Verification items for the finished model (mm, model axes). Face numbers are marked on the shaded views. A direction names the side the tool comes from. Coordinates: 2 decimals unless noted, no trailing zeros. Order: outer loops, then holes, each group sorted by start corner. A loop starts at its lowest first (then second) coordinate and runs counter-clockwise, first axis right, second up. Notation, with made-up numbers: (62.5, 56) -> (94.5, 56) arc R17 ccw to (94.5, 81) -> close; hole circle Ø10 at (-22, -14.5). An arc over 180 degrees is marked (long way). Answer as CSV lines item,"result".
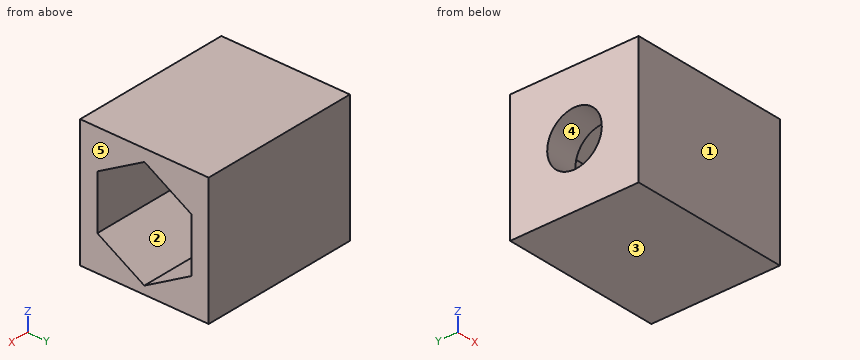
```python
from build123d import *

# Parameters (mm, degrees)
CYLINDER031_R              = 1.7
CYLINDER031_DEPTH          = 20
EXTRUDE004_DEPTH           = 9
EXTRUDE004_PLACEMENT_ANGLE = 90
BOX042_W                   = 10
BOX042_H                   = 8
BOX042_DEPTH               = 8


with BuildPart() as cylinder031:
    # Cylinder031 → Cylinder031 (new body)
    with BuildSketch(Plane(origin=(140, 9.74, 51.5), x_dir=(0, 0, -1), z_dir=(1, 0, 0))):
        Circle(CYLINDER031_R)
    extrude(amount=CYLINDER031_DEPTH)


with BuildPart() as extrude004:
    # Sketch004 → Extrude004 (new body)
    with BuildSketch(Plane.XY.offset(75)):
        Polygon((-29.694611, 6.813304), (-28.00073, 9.738351), (-29.686954, 12.667818), (-33.06706, 12.672239), (-34.760941, 9.747192), (-33.074716, 6.817725), align=None)
    extrude(amount=EXTRUDE004_DEPTH)


with BuildPart() as extrude004_1:
    # Extrude004 placement: moved
    add(extrude004.part.moved(Location((71, 0, 0))).rotate(Axis((71, 0, 0), (0, 1, 0)), EXTRUDE004_PLACEMENT_ANGLE))


with BuildPart() as cut050:
    # Box042 → Box042 (new body)
    with BuildSketch(Plane(origin=(144, 5.745, 27.5), x_dir=(1, 0, 0), z_dir=(0, 0, 1))):
        with Locations((5, 4)):
            Rectangle(BOX042_W, BOX042_H)
    extrude(amount=BOX042_DEPTH)

    # Cut049: cut Extrude004
    add(extrude004_1.part, mode=Mode.SUBTRACT)


with BuildPart() as cut050_1:
    # Cut049 placement: moved
    add(cut050.part.moved(Location((0, 0, 20))))

    # Cut050: cut Cylinder031
    add(cylinder031.part, mode=Mode.SUBTRACT)


solid = cut050_1.part
```
Item 1: Tool access check on the marked faces 1 and 2. Record the directions out of +Z, -Z, +X, -X, +Y, -Y that give a thin tool (end or side, any length) a straight path to the whole face; none if there is none.
Answer list:
face 1,"+Z, -Z, +X, -X, -Y"
face 2,"+X"
Item 2: Release check for a two-part mould opening along Z. For the marked faces 3, 4 and 5 record: +Z half, -Z half, draft (parallel to the pull), parting line (faces both ways), or undercut.
Answer list:
face 3,"-Z half"
face 4,"undercut"
face 5,"draft"
Item 3: Section check D-D, the plane z = 54. Record the boundary of the cut face in (x, y) (3 decimals), plus the area to 3 significant figures.
Answer list:
outline,"(144, 5.745) -> (154, 5.745) -> (154, 8.425) -> (146, 8.425) -> (146, 11.061) -> (154, 11.061) -> (154, 13.745) -> (144, 13.745) -> close"
area,"58.9 mm2"
Item 4: Section check B-B, the plane x = 145. Record the boundary of the cut face in (y, z) (3 decimals), plus the area to 3 significant figures.
Answer list:
outline,"(5.745, 47.5) -> (13.745, 47.5) -> (13.745, 55.5) -> (5.745, 55.5) -> close; hole circle Ø3.4 at (9.74, 51.5)"
area,"54.9 mm2"
Item 5: Section check C-C, the plane y = 10.5. Record the boundary of the cut face in (x, z) (3 decimals), plus the area to 3 significant figures.
Answer list:
outline,"(144, 47.5) -> (154, 47.5) -> (154, 48.439) -> (146, 48.439) -> (146, 49.979) -> (144, 49.979) -> close; (144, 53.021) -> (146, 53.021) -> (146, 54.325) -> (154, 54.325) -> (154, 55.5) -> (144, 55.5) -> close"
area,"26.8 mm2"
Item 6: Depth check by flat-ended pin: pin 1 Ø1.5 at (y, z) = (11.5, 50) entering from +X. Enter the tip coordinate at first touch or a pass-through.
Answer list:
pin 1,"x = 146"
Item 7: Section check A-A, the plane z = 52.5. Record the boundary of the cut face in (x, y) (1 decimal).
Answer list:
outline,"(144, 5.7) -> (154, 5.7) -> (154, 6.8) -> (146, 6.8) -> (146, 8.4) -> (144, 8.4) -> close; (144, 11.1) -> (146, 11.1) -> (146, 12.7) -> (154, 12.7) -> (154, 13.7) -> (144, 13.7) -> close"
Item 8: Thickness scan on line 1 (Y direction, x = 145.3, z = 51.5) (3 decimals); line 2 (Y direction, x = 146.75, z = 52.75) (3 decimals); line 3 (Z direction, x = 144.8, y = 9.74). Record the ranges inside material, lowest first.
Answer list:
line 1,"5.745 to 8.04, 11.44 to 13.745"
line 2,"5.745 to 6.817, 12.672 to 13.745"
line 3,"47.5 to 49.8, 53.2 to 55.5"
